Verification items for the finished model (mm, model axes). A direction names the side the tool comes from. Give positions to 0.01 mm unless a question says otherwise; leave off trailing zeros. Order: outer loops, then holes, each group sorted by start corner. A loop starts at its lowest first (then second) coordinate and runs counter-clockwise, first axis right, second up. Notation, with made-up numbers: (57.25, 51) - (90.25, 51) arc R6 cw to (90.25, 56) - close; hole circle Ø7 at (84, -34.5). An arc over 180 degrees is marked (long way). Answer as a JSON object with one key per item and string values.
```python
from build123d import *

# Parameters (mm, degrees)
F0_W     = 5
F0_H     = 5
F1_DEPTH = 4
F2_R     = 1
F3_DEPTH = 2
F4_W     = 5
F4_H     = 24.4
F4_H_2   = 5
F5_DEPTH = 3
F7_DEPTH = 25


with BuildPart() as f1:
    # F0 (on Front) → F1 (new body)
    with BuildSketch(Plane.XZ):
        Rectangle(F0_W, F0_H)
    extrude(amount=F1_DEPTH)

    # F2 (on face) → F3 (join)
    with BuildSketch(Plane.XZ.offset(4)):
        Circle(F2_R)
    extrude(amount=F3_DEPTH)

    # F4 (on face) → F5 (join)
    with BuildSketch(Plane(origin=(0, 0, 0), x_dir=(-1, 0, 0), z_dir=(0, 1, 0))):
        with Locations((0, -14.7)):
            Rectangle(F4_W, F4_H)
        Rectangle(F4_W, F4_H_2)
    extrude(amount=F5_DEPTH)

    # F6 (on face) → F7 (join)
    with BuildSketch(Plane(origin=(0, 0, -26.9), x_dir=(1, 0, 0), z_dir=(0, 0, -1))):
        with BuildLine():
            Line((-2.5, 0), (0, 0))
            Line((0, 0), (2.5, 0))
            Line((2.5, 0), (2.5, -2.5383484153))
            ThreePointArc((2.5, -2.5383484153), (5.7662812973, 0.0313730334), (7, 4))
            ThreePointArc((7, 4), (-3.9686269666, 9.7662812973), (-2.5, -2.5383484153))
            Line((-2.5, -2.5383484153), (-2.5, 0))
        make_face()
        with BuildLine():
            ThreePointArc((0, 0), (-2.8284271247, 6.8284271247), (4, 4))
            ThreePointArc((4, 4), (2.8284271247, 1.1715728753), (0, 0))
        make_face(mode=Mode.SUBTRACT)
        with BuildLine():
            Line((2.5, 0), (0, 0))
            Line((0, 0), (-2.5, 0))
            Line((-2.5, 0), (-2.5, -2.5383484153))
            ThreePointArc((-2.5, -2.5383484153), (-1.2711335675, -2.8836196477), (0, -3))
            ThreePointArc((0, -3), (1.2711335675, -2.8836196477), (2.5, -2.5383484153))
            Line((2.5, -2.5383484153), (2.5, 0))
        make_face()
    extrude(amount=F7_DEPTH)


solid = f1.part
```
(1) Access from +Z, -Z, +X, -X, +Y, -Y to the whole of each face (thin tool, end or side, straight path). Record for faces 4 (the flat face through (-2.5, 1, -12)), 5 (the flat face through (-0.03, -4, 1.15)), 6 (the flat face through (2.5, 1, -9)).
Computed values:
{"face 4": "+Z, -X, +Y, -Y", "face 5": "-Y", "face 6": "+Z, +X, +Y, -Y"}
(2) Section check C-C (x = 3). Record the cut outline in (y, z), then the cut area to 3 significant figures.
Computed values:
{"outline": "(-10.32, -51.9) - (-6.65, -51.9) - (-6.65, -26.9) - (-10.32, -26.9) - close; (-1.35, -51.9) - (2.32, -51.9) - (2.32, -26.9) - (-1.35, -26.9) - close", "area": "184 mm²"}
(3) Section check A-A (z = 0). Record the cut outline in (x, y), then the cut area to 3 significant figures.
Computed values:
{"outline": "(-2.5, -4) - (-1, -4) - (-1, -6) - (1, -6) - (1, -4) - (2.5, -4) - (2.5, 3) - (-2.5, 3) - close", "area": "39.0 mm²"}
(4) Section check D-D (z = -43.5). Record the cut outline in (x, y), then the cut area to 3 significant figures.
Computed values:
{"outline": "circle Ø14 at (0, -4); hole circle Ø8 at (0, -4)", "area": "104 mm²"}
(5) Section check B-B (y = -6.5). Record the cut outline in (x, z), then the cut area to 3 significant figures.
Computed values:
{"outline": "(-6.54, -51.9) - (-3.12, -51.9) - (-3.12, -26.9) - (-6.54, -26.9) - close; (3.12, -51.9) - (6.54, -51.9) - (6.54, -26.9) - (3.12, -26.9) - close", "area": "171 mm²"}
(6) Gauge pin test, flat ends, axial feed: pin 1 Ø2 at (x, y) = (-1, -3) entering from -Z; pin 2 Ø7.5 at (y, z) = (-1, -9.5) entering from +X; pin 3 Ø1.5 at (x, z) = (0, -11) entering from -Y. Record the tip position at first contact, or that the pin passes through.
Computed values:
{"pin 1": "stops at z = -2.5", "pin 2": "stops at x = 2.5", "pin 3": "stops at y = 0"}
(7) Material ranges on line 1 along X through (y, z) = (-4, -36); line 2 along Y through (x, z) = (0.5, -1.5); line 3 along Z through (x, y) = (-1.5, -1.5), recorded low to high. Write a range as [from, to].
Computed values:
{"line 1": "x = [-7, -4], [4, 7]", "line 2": "y = [-4, 3]", "line 3": "z = [-2.5, 2.5]"}
(8) Release check for a two-part mould opening along Z. For faces 1 (the flat face through (0, 0, -15)), 2 (the flat face through (0, -6, 0)), 3 (the flat face through (3, -1, -51.9)) record: pulls with the +Z half, pulls with the -Z half, needs draft (parallel to the pull), parting line crosses it, or undercut.
Computed values:
{"face 1": "undercut", "face 2": "needs draft", "face 3": "pulls with the -Z half"}
